```python
from build123d import *

# Parameters (mm, degrees)
F0_W     = 105
F0_H     = 60
F1_DEPTH = 20
F2_R     = 7.5
F3_DEPTH = 68.6
F4_DEPTH = 55.5
F5_R     = 2.5


with BuildPart() as f1:
    # F0 (on Top) → F1 (new body)
    with BuildSketch(Plane.XY):
        Rectangle(F0_W, F0_H)
    extrude(amount=-F1_DEPTH)

    # F2 (on face) → F3 (cut)
    with BuildSketch(Plane.XY):
        with BuildLine():
            ThreePointArc((-7.5, 0), (0, -7.5), (7.5, 0))
            ThreePointArc((7.5, 0), (0, 7.5), (-7.5, 0))
        make_face()
        with Locations((-22.5, 0)):
            Circle(F2_R)
        with BuildLine():
            ThreePointArc((30, 0), (22.5, 7.5), (15, 0))
            ThreePointArc((15, 0), (22.5, -7.5), (30, 0))
        make_face()
    extrude(amount=-F3_DEPTH, mode=Mode.SUBTRACT)

    # F2 (on face) → F4 (cut)
    with BuildSketch(Plane.XY):
        with BuildLine():
            ThreePointArc((-7.5, 0), (0, -7.5), (7.5, 0))
            ThreePointArc((7.5, 0), (0, 7.5), (-7.5, 0))
        make_face()
        with Locations((-22.5, 0)):
            Circle(F2_R)
        with BuildLine():
            ThreePointArc((30, 0), (22.5, 7.5), (15, 0))
            ThreePointArc((15, 0), (22.5, -7.5), (30, 0))
        make_face()
    extrude(amount=-F4_DEPTH, mode=Mode.SUBTRACT)

    # F5
    f5_edges = [f1.edges().sort_by_distance(p)[0] for p in [
        (0, -30, 0),
        (52.5, 0, 0),
        (52.5, 0, -20),
        (52.5, -30, -10),
        (0, -30, -20),
        (-52.5, -30, -10),
        (-52.5, 0, 0),
        (-52.5, 0, -20),
        (0, 30, 0),
        (0, 30, -20),
    ]]
    fillet(f5_edges, radius=F5_R)


solid = f1.part
```
Work out the finished part from the listing and answer in its coordinate system (mm). Give positions to 0.01 mm unless a question says otherwise; leave off trailing zeros. Loops run counter-clockwise (first coordinate to the right, second up) from the corner with the lowest first, then second, coordinate; pieces in that order, holes last. Notation, with made-up numbers: M -38,-6.75 L 13,-6.75 A10 cw 13,10.25 Z; hole C 48.25,45 d8. An arc over 180 degrees is marked long. One line per item, written item: value. Start each with the question number.
1. Find section D-D (x = 1.5). Give the vertices of the cut face in (y, z), and give its area (3 significant figures).
2. Find the intervals of material crossed by probe 1 along Y at (x, z) = (22.5, -12.5); probe 2 along X at (y, z) = (0.5, -4.5); probe 3 along X at (y, z) = (-3, -3.75), in increasing order.
3. Determine the mould class of faces 1 (the face through (30, 0, -10)), 2 (the face through (0.735, 29.287, -0.752)), 3 (the face through (-52.5, 1, -10)) for opening direction Y: released by +Y, released by -Y, zero draft, split by the parting line, or undercut.
4. Find section C-C (x = -22.5). Give the vertices of the cut face in (y, z).
5. This flat-tipped pin is pushed along its axis until it touches: P1, Ø12, axis at x = -22.5, y = 0, coming from the +Z side. Where does it stop, or does it pass through?
6. Find section B-B (z = -16.5). Give the vertices of the cut face in (x, y).
7. Find section A-A (y = 0). Give the vertices of the cut face in (x, z).
Reported:
1. outline: M -30,-17.5 A2.5 ccw -27.5,-20 L -7.35,-20 L -7.35,0 L -27.5,0 A2.5 ccw -30,-2.5 Z; M 7.35,-20 L 27.5,-20 A2.5 ccw 30,-17.5 L 30,-2.5 A2.5 ccw 27.5,0 L 7.35,0 Z
1. area: 901 mm²
2. probe 1: y = -30 to -7.5, 7.5 to 30
2. probe 2: x = -52.5 to -29.98, -15.02 to -7.48, 7.48 to 15.02, 29.98 to 52.5
2. probe 3: x = -52.5 to -29.37, -15.63 to -6.87, 6.87 to 15.63, 29.37 to 52.5
3. face 1: undercut
3. face 2: released by +Y
3. face 3: zero draft
4. outline: M -30,-17.5 A2.5 ccw -27.5,-20 L -7.5,-20 L -7.5,0 L -27.5,0 A2.5 ccw -30,-2.5 Z; M 7.5,-20 L 27.5,-20 A2.5 ccw 30,-17.5 L 30,-2.5 A2.5 ccw 27.5,0 L 7.5,0 Z
5. P1: passes through
6. outline: M -52.5,-27.5 A2.5 ccw -50,-30 L 50,-30 A2.5 ccw 52.5,-27.5 L 52.5,30 L -52.5,30 Z; hole C -22.5,0 d15; hole C 0,0 d15; hole C 22.5,0 d15
7. outline: M -52.5,-17.5 A2.5 ccw -50,-20 L -30,-20 L -30,0 L -50,0 A2.5 ccw -52.5,-2.5 Z; M -15,-20 L -7.5,-20 L -7.5,0 L -15,0 Z; M 7.5,-20 L 15,-20 L 15,0 L 7.5,0 Z; M 30,-20 L 50,-20 A2.5 ccw 52.5,-17.5 L 52.5,-2.5 A2.5 ccw 50,0 L 30,0 Z
